Job drawing, mm, ordinate dimensions from the low corner. One solid piece. Give positions to 0.01 mm unless a question says otherwise; leave off trailing zeros. Order: outer loops, then holes, each group sorted by start corner. A loop starts at its lowest first (then second) coordinate and runs counter-clockwise, first axis right, second up.
Item 1: Band-saw the part on A-A on z = 6.5. Give the cut face in (x, y).
Item 2: Band-saw the part on B-B on x = 186. Give the cut face in (y, z), plus the area to 3 significant figures.
Item 3: Wall check: L1, parallel to Y at x = 60, z = 3.5; L2, parallel to X at y = 8, z = 5.75. Give the ranges that are in metal, low to high.
Item 4: Flat gauge pin, fed straight in: P1, Ø2, axis at x = 194.5, z = 3, coming from the -Y side. Where does the tip first touch, or does it go through?
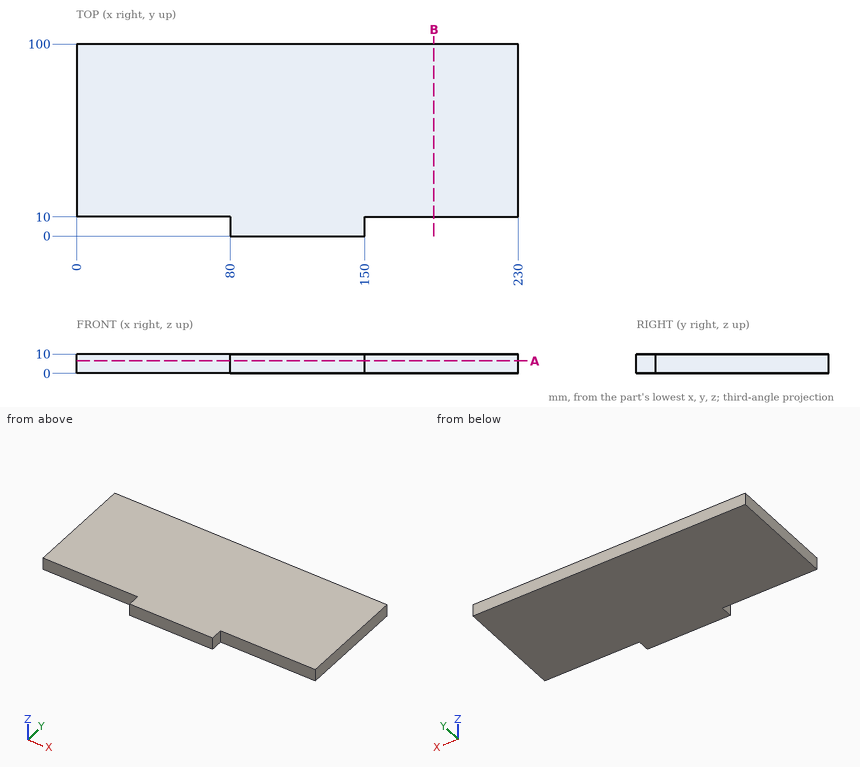
The answers:
1. outline: (0, 10) - (80, 10) - (80, 0) - (150, 0) - (150, 10) - (230, 10) - (230, 100) - (0, 100) - close
2. outline: (10, 0) - (100, 0) - (100, 10) - (10, 10) - close
2. area: 900 mm2
3. L1: y = 10 to 100
3. L2: x = 80 to 150
4. P1: stops at y = 10
